Source: CAD feature listing. Evaluate the final solid. Frame: model axes, mm. Face numbers are marked on the shaded views. A direction names the side the tool comes from. Give positions to 0.01 mm unless a question says otherwise; leave off trailing zeros. Order: outer loops, then holes, each group sorted by start corner. A loop starts at its lowest first (then second) coordinate and runs counter-clockwise, first axis right, second up. Notation, with made-up numbers: M 45.5,26 L 82.5,26 A17 cw 82.5,57 Z; hole C -14,83.25 d9. An arc over 180 degrees is marked long. Answer in a Markdown table with one row per item. Add a question column.
(1) Section query B-B, the plane z = 0. Return loops of the section in (x, y).
(2) Pin query (flat end, axial travel): P1, Ø11, axis at x = 0, z = 0, coming from the -Y side; P2, Ø2, axis at y = -5.5, z = -10.5, coming from the +X side; P3, Ø4, axis at y = -1, z = -8, coming from the -X side; P4, Ø6, axis at x = 15, z = 11.5, coming from the +Y side. Return the tip coordinate at first contact, or that it passes through.
(3) Set-up query: the marked faces 4, 5 and 6. Return all of +Z, -Z, +X, -X, +Y, -Y with unobstructed straight access to the full face (end or side cutting, diameter ignored); none if empty.
(4) Material intervals for line 1 along X through (y, z) = (3.5, 0); line 2 along Y through (x, z) = (-8.5, 17); line 3 along Y through (x, z) = (0, -11.1), sorted ascending.
(5) Section query C-C, the plane y = -8.5. Return loops of the section in (x, z).
(6) Mould query, pull axis Y, two halves, no side actions, for the marked faces 1, 2 and 3. Classes: pulls with the +Y half, pulls with the -Y half, needs draft (parallel to the pull), parting line crosses it, or undercut.
(7) Section query D-D, the plane x = -17. Return loops of the section in (y, z).
(8) Section query A-A, the plane x = 0. Return loops of the section in (y, z).
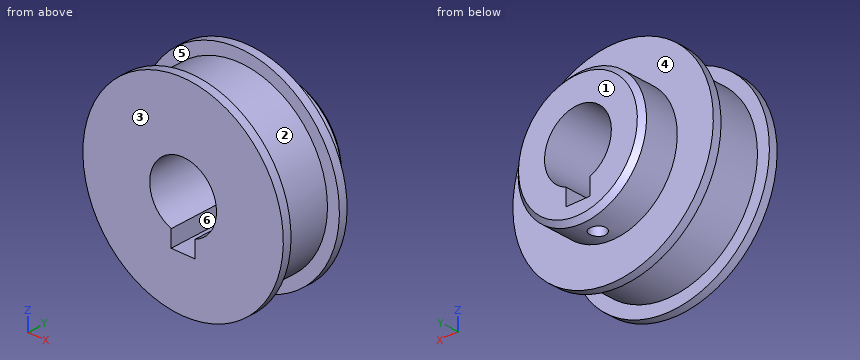
from build123d import *

# Parameters (mm, degrees)
SMUSSO1_SIZE             = 1
SCHIZZO2_R               = 6
TAGLIO_ESTRUSIONE1_DEPTH = 38.259227045
SCHIZZO3_R               = 1.65
TAGLIO_ESTRUSIONE2_DEPTH = 32.75787304
SCHIZZO4_R               = 7
TAGLIO_ESTRUSIONE3_DEPTH = 38.259227106
SCHIZZO5_W               = 5
SCHIZZO5_H               = 6
TAGLIO_ESTRUSIONE4_DEPTH = 38.259227106


with BuildPart() as part:
    # Schizzo1 → Rivoluzione1 (revolve)
    with BuildSketch(Plane.XY, mode=Mode.PRIVATE) as rivoluzione1_sk:
        Polygon((0, 11.25), (13.45, 11.25), (13.45, 3.25), (21, 3.25), (21, 1.5), (18.5, 1.5), (18.5, -9.5), (21, -9.5), (21, -11.25), (0, -11.25), align=None)
    revolve(rivoluzione1_sk.sketch.rotate(Axis((0, -12.375, 0), (0, 1, 0)), 90), axis=Axis((0, -12.375, 0), (0, 1, 0)))

    # Smusso1
    smusso1_edges = [part.edges().sort_by_distance(p)[0] for p in [
        (0, 11.25, 13.45),
    ]]
    chamfer(smusso1_edges, length=SMUSSO1_SIZE)

    # Schizzo2 → Taglio-Estrusione1 (cut, through all)
    with BuildSketch(Plane(origin=(0, 11.25, 0), x_dir=(1, 0, 0), z_dir=(0, 1, 0))):
        with Locations(Location((0, 0, 0), (0, 0, 270))):
            Circle(SCHIZZO2_R)
    extrude(amount=-TAGLIO_ESTRUSIONE1_DEPTH, mode=Mode.SUBTRACT)

    # Schizzo3 → Taglio-Estrusione2 (cut, through all)
    with BuildSketch(Plane.XY):
        with Locations((0, 6.75)):
            Circle(SCHIZZO3_R)
    extrude(amount=-TAGLIO_ESTRUSIONE2_DEPTH, mode=Mode.SUBTRACT)

    # Schizzo4 → Taglio-Estrusione3 (cut, through all)
    with BuildSketch(Plane(origin=(0, 11.25, 0), x_dir=(1, 0, 0), z_dir=(0, 1, 0))):
        with Locations(Location((0, 0, 0), (0, 0, 270))):
            Circle(SCHIZZO4_R)
    extrude(amount=-TAGLIO_ESTRUSIONE3_DEPTH, mode=Mode.SUBTRACT)

    # Schizzo5 → Taglio-Estrusione4 (cut, through all)
    with BuildSketch(Plane(origin=(0, 11.25, 0), x_dir=(1, 0, 0), z_dir=(0, 1, 0))):
        with Locations((0, 7)):
            Rectangle(SCHIZZO5_W, SCHIZZO5_H)
    extrude(amount=-TAGLIO_ESTRUSIONE4_DEPTH, mode=Mode.SUBTRACT)


solid = part.part
Values follow:
| question | item | result |
|---|---|---|
| 1 | outline | M -21,-11.25 L -7,-11.25 L -7,11.25 L -12.45,11.25 L -13.45,10.25 L -13.45,3.25 L -21,3.25 L -21,1.5 L -18.5,1.5 L -18.5,-9.5 L -21,-9.5 Z; M 7,-11.25 L 21,-11.25 L 21,-9.5 L 18.5,-9.5 L 18.5,1.5 L 21,1.5 L 21,3.25 L 13.45,3.25 L 13.45,10.25 L 12.45,11.25 L 7,11.25 Z |
| 2 | P1 | passes through |
| 2 | P2 | stops at x = 15.87 |
| 2 | P3 | stops at x = -17.5 |
| 2 | P4 | stops at y = 3.25 |
| 3 | face 4 | +Y |
| 3 | face 5 | none |
| 3 | face 6 | +Y, -Y |
| 4 | line 1 | x = -13.45 to -7, 7 to 13.45 |
| 4 | line 2 | y = -11.25 to -9.5, 1.5 to 3.25 |
| 4 | line 3 | y = -11.25 to 5.1, 8.4 to 11.25 |
| 5 | outline | C 0,0 d37; hole M -2.5,-10 L 2.5,-10 L 2.5,-6.54 A7 ccw long -2.5,-6.54 Z |
| 6 | face 1 | pulls with the +Y half |
| 6 | face 2 | undercut |
| 6 | face 3 | pulls with the -Y half |
| 7 | outline | M -11.25,-12.33 L -9.5,-12.33 L -9.5,-7.3 L 1.5,-7.3 L 1.5,-12.33 L 3.25,-12.33 L 3.25,12.33 L 1.5,12.33 L 1.5,7.3 L -9.5,7.3 L -9.5,12.33 L -11.25,12.33 Z |
| 8 | outline | M -11.25,-21 L -9.5,-21 L -9.5,-18.5 L 1.5,-18.5 L 1.5,-21 L 3.25,-21 L 3.25,-13.45 L 5.1,-13.45 L 5.1,-10 L -11.25,-10 Z; M -11.25,7 L 11.25,7 L 11.25,12.45 L 10.25,13.45 L 3.25,13.45 L 3.25,21 L 1.5,21 L 1.5,18.5 L -9.5,18.5 L -9.5,21 L -11.25,21 Z; M 8.4,-13.45 L 10.25,-13.45 L 11.25,-12.45 L 11.25,-10 L 8.4,-10 Z |
